```python
from build123d import *

# Parameters (mm, degrees)
BASEHEAD_DEPTH = 7.5
SKETCH4_W      = 0.5
SKETCH4_H      = 12.092304845


# Read off the part's stored shape, not the designer's step: HeadChamfer
with BuildPart() as part:
    # Sketch1 → BaseHead (new body)
    with BuildSketch(Plane(origin=(0, 0, 0), x_dir=(0, 0, -1), z_dir=(1, 0, 0))):
        Polygon((9, 5.196152423), (9, -5.196152423), (0, -10.392304845), (-9, -5.196152423), (-9, 5.196152423), (0, 10.392304845), align=None)
    extrude(amount=BASEHEAD_DEPTH)

    # HeadChamfer outline → HeadChamfer (revolve, cut)
    with BuildSketch(Plane.YX):
        Polygon((10.392304847, 0.803847578), (9, 0), (10.392304847, 0), align=None)
    revolve(axis=Axis((0, 0, 0), (1, 0, 0)), mode=Mode.SUBTRACT)

    # HeadChamfer 2 outline → HeadChamfer 2 (revolve)
    with BuildSketch(Plane.YX):
        Polygon((6, 7.5), (6, 41.536), (5.036, 42.5), (0, 42.5), (0, 7.5), align=None)
    revolve(axis=Axis((0, 0, 0), (1, 0, 0)))

    # Sketch4 → BearingFace (revolve, cut)
    with BuildSketch(Plane.XY, mode=Mode.PRIVATE) as bearingface_sk:
        with Locations((7.25, 14.346152423)):
            Rectangle(SKETCH4_W, SKETCH4_H)
    revolve(bearingface_sk.sketch.rotate(Axis((0, 0, 0), (1, 0, 0)), 90), axis=Axis((0, 0, 0), (1, 0, 0)), mode=Mode.SUBTRACT)


solid = part.part
```
Geometry check sheet. Reference: the model listing, model coordinates, mm. A direction names the side the tool comes from. Round coordinates to 2 decimals unless told otherwise and drop trailing zeros. Write each loop counter-clockwise with the first axis right and the second up, starting at its lowest first coordinate (ties: lowest second). Pieces come first, ordered by that corner, then holes. Notation, with made-up numbers: (68.25, 36) - (108.25, 36) arc R33 cw to (108.25, 66) - close; hole circle Ø6 at (66, 87). An arc over 180 degrees is marked (long way). Write each question's results on one line, items separated by ' | '.
(1) Sectioned sample at A-A, the plane x = 20.5. Enter the section's corners in (y, z).
Computed:
outline: circle Ø12 at (0, 0)
(2) Thickness scan on probe 1 along Y at (x, z) = (16, -3.25); probe 2 along X at (y, z) = (6.5, -1); probe 3 along X at (y, z) = (-1.5, 8.25). Record the ranges inside material, lowest first. Write a range as from..to.
Computed:
probe 1: y = -5.04..5.04 | probe 2: x = 0..7.5 | probe 3: x = 0..7
(3) Set-up check for faces 1 (the face through (0.19, -9.33, 0.02)), 2 (the face through (25, -6, 0)): record each of +Z, -Z, +X, -X, +Y, -Y from which the full face is reachable in a straight line by a thin tool's end or side.
Computed:
face 1: -X, -Y | face 2: +X
(4) Depth check by flat-ended pin: pin 1 Ø8 at (x, y) = (22, -0.5) entering from +Z; pin 2 Ø3 at (x, z) = (29, -2) entering from -Y; pin 3 Ø5 at (x, y) = (32, 4.5) entering from -Z; pin 4 Ø10 at (y, z) = (-8, 4.5) entering from +X. Enter the tip coordinate at first touch or a pass-through.
Computed:
pin 1: stops at z = 6 | pin 2: stops at y = -5.98 | pin 3: stops at z = -5.66 | pin 4: stops at x = 42.5
